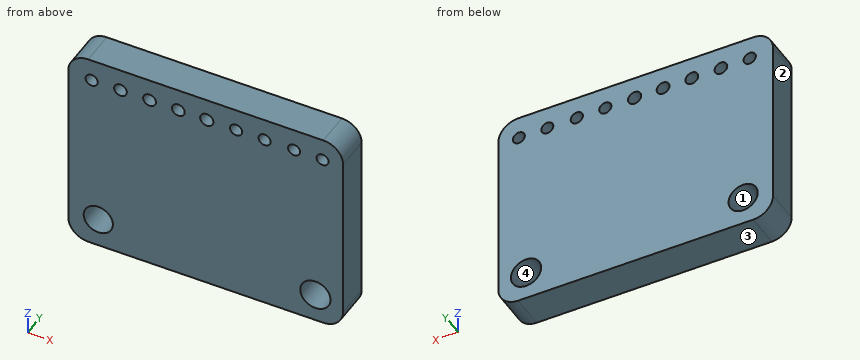
```python
from build123d import *

# Parameters (mm, degrees)
SKETCH1_W           = 25
SKETCH1_H           = 19
BOSS_EXTRUDE1_DEPTH = 3.14
SKETCH2_R           = 1.328703157
CUT_EXTRUDE1_DEPTH  = 32.557243226
SKETCH3_R           = 1.379079597
CUT_EXTRUDE2_DEPTH  = 32.557243226
SKETCH4_R           = 0.546420727
SKETCH4_R_2         = 0.547156774
SKETCH4_R_3         = 0.553895188
SKETCH4_R_4         = 0.554442322
SKETCH4_R_5         = 0.60258245
SKETCH4_R_6         = 0.580608074
SKETCH4_R_7         = 0.583065552
SKETCH4_R_8         = 0.578153998
SKETCH4_R_9         = 0.55656492
CUT_EXTRUDE3_DEPTH  = 32.557243226
FILLET1_R           = 1.8


with BuildPart() as part:
    # Sketch1 → Boss-Extrude1 (new body)
    with BuildSketch(Plane(origin=(0, 0, 0), x_dir=(1, 0, 0), z_dir=(0, 1, 0))):
        with Locations((12.5, 9.5)):
            Rectangle(SKETCH1_W, SKETCH1_H)
    extrude(amount=BOSS_EXTRUDE1_DEPTH)

    # Sketch2 → Cut-Extrude1 (cut, through all)
    with BuildSketch(Plane(origin=(0, 3.14, 0), x_dir=(1, 0, 0), z_dir=(0, 1, 0))):
        with Locations(Location((2.722594634, 16.331436322, 0), (0, 0, 270))):
            Circle(SKETCH2_R)
    extrude(amount=-CUT_EXTRUDE1_DEPTH, mode=Mode.SUBTRACT)

    # Sketch3 → Cut-Extrude2 (cut, through all)
    with BuildSketch(Plane(origin=(0, 3.14, 0), x_dir=(1, 0, 0), z_dir=(0, 1, 0))):
        with Locations(Location((22.483739106, 16.364797794, 0), (0, 0, 270))):
            Circle(SKETCH3_R)
    extrude(amount=-CUT_EXTRUDE2_DEPTH, mode=Mode.SUBTRACT)

    # Sketch4 → Cut-Extrude3 (cut, through all)
    with BuildSketch(Plane(origin=(0, 3.14, 0), x_dir=(1, 0, 0), z_dir=(0, 1, 0))):
        with Locations(Location((23.137145161, 2.05046074, 0), (0, 0, 270))):
            Circle(SKETCH4_R)
        with Locations(Location((20.543630063, 2.05046074, 0), (0, 0, 270))):
            Circle(SKETCH4_R_2)
        with Locations(Location((17.860899334, 2.05046074, 0), (0, 0, 270))):
            Circle(SKETCH4_R_3)
        with Locations(Location((15.268099294, 2.05046074, 0), (0, 0, 270))):
            Circle(SKETCH4_R_4)
        with Locations(Location((12.597553851, 2.05046074, 0), (0, 0, 270))):
            Circle(SKETCH4_R_5)
        with Locations(Location((10.010026119, 2.05046074, 0), (0, 0, 270))):
            Circle(SKETCH4_R_6)
        with Locations(Location((7.390364783, 2.05046074, 0), (0, 0, 270))):
            Circle(SKETCH4_R_7)
        with Locations(Location((4.744820308, 2.05046074, 0), (0, 0, 270))):
            Circle(SKETCH4_R_8)
        with Locations(Location((2.121365988, 2.05046074, 0), (0, 0, 270))):
            Circle(SKETCH4_R_9)
    extrude(amount=-CUT_EXTRUDE3_DEPTH, mode=Mode.SUBTRACT)

    # Fillet1
    fillet1_edges = [part.edges().sort_by_distance(p)[0] for p in [
        (0, 1.57, -19),
        (25, 1.57, -19),
        (25, 1.57, 0),
        (0, 1.57, 0),
    ]]
    fillet(fillet1_edges, radius=FILLET1_R)


solid = part.part
```
Input: part model. Units: mm. Frame: model coordinates. Face numbers are marked on the shaded views. Give positions to 0.01 mm unless a question says otherwise; leave off trailing zeros. Loops run counter-clockwise (first coordinate to the right, second up) from the corner with the lowest first, then second, coordinate; pieces in that order, holes last. Notation, with made-up numbers: (62, 68) -> (70, 68) arc R25 ccw to (70, 87) -> close; hole circle Ø3 at (76.25, -3.75). An arc over 180 degrees is marked (long way). Use a Markdown table: item, result.
Q1. Section query B-B, the plane y = 0.3. State how many separate pieces and enclosed holes the cut face has, plus the area to 3 significant figures.
Entries:
| item | result |
|---|---|
| separate pieces | 1 |
| enclosed holes | 11 |
| area | 452 mm² |
Q2. Section query A-A, the plane z = -15.5. Return the cut outline in (x, y), plus the area to 3 significant figures.
Entries:
| item | result |
|---|---|
| outline | (0, 0) -> (1.69, 0) -> (1.69, 3.14) -> (0, 3.14) -> close; (3.76, 0) -> (21.41, 0) -> (21.41, 3.14) -> (3.76, 3.14) -> close; (23.56, 0) -> (25, 0) -> (25, 3.14) -> (23.56, 3.14) -> close |
| area | 65.2 mm² |
Q3. First-contact query: P1, Ø0.9, axis at x = 7.39, z = -2.05, coming from the +Y side (3 decimals). Flat tip, straight axial feed; report the tip coordinate or a pass-through.
Entries:
| item | result |
|---|---|
| P1 | passes through |
Q4. Pull-direction query (X, two-part tool) for the marked faces 1, 2, 3 and 4; classes: pulls with the +X half, pulls with the -X half, needs draft (parallel to the pull), parting line crosses it, or undercut.
Entries:
| item | result |
|---|---|
| face 1 | undercut |
| face 2 | pulls with the -X half |
| face 3 | needs draft |
| face 4 | undercut |
Q5. Ray query, probe 1 along X at (y, z) = (2.3, -17); probe 2 along X at (y, z) = (2.7, -15.25); probe 3 along Z at (x, y) = (23.5, 1.5). Return the intervals inside material, ascending. Write a range as from..to.
Entries:
| item | result |
|---|---|
| probe 1 | x = 0..1.57, 3.87..21.26, 23.71..25 |
| probe 2 | x = 0..1.95, 3.49..21.67, 23.3..25 |
| probe 3 | z = -18.97..-17.3, -15.43..-2.46, -1.64..-0.03 |
